Can you work these out from the model? Positions are in its coordinate system, mm. A direction names the side the tool comes from. Coordinates: 2 decimals unless noted, no trailing zeros. Order: outer loops, then holes, each group sorted by start corner. A loop starts at its lowest first (then second) coordinate and runs counter-clockwise, first axis right, second up. Notation, with made-up numbers: (-3, 5) -> (8, 5) arc R6 ccw to (8, 13) -> close; hole circle Ø3 at (51.25, -34.75). An arc over 180 degrees is marked (long way). Write item = value, one per line.
Autodesk Inventor part; units mm, degrees
ref_plane "YZ Plane" through (0, 0, 0) normal (1, 0, 0) x (0, 1, 0)
ref_plane "XZ Plane" through (0, 0, 0) normal (0, 1, 0) x (-1, 0, 0)
ref_plane "XY Plane" through (0, 0, 0) normal (0, 0, 1) x (1, 0, 0)
sketch "Base" plane through (0, 0, 0) normal (0, 1, 0) x (-1, 0, 0)
  line L0 (0, 0) -> (-12, 0)
  line L1 (-12, 0) -> (-12, -11.4)
  line L2 (-12, -11.4) -> (0, -11.4) construction
  line L3 (0, -11.4) -> (0, 0)
  circle A0 centre (-3.175, -3.175) radius 3.175
  circle A1 centre (-6.5, -11.4) radius 6.5
  line L4 (-6.5, -4.9) -> (-6.5, 0)
  line L5 (-6.5, -4.9) -> (-12, -4.9)
  line L6 (-9.25, -4.9) -> (-9.25, 0)
  point P0 (0, 0)
  point P1 (-12, -7.9359)
  dimension "d24" = 13
  dimension "d21" = 12
  dimension "d22" = 11.4
  dimension "d23" = 6.35
  dimension "d26" = 5.5
  dimension "d36" = 5.5
extrude "Stock" add sketch "Base" against normal blind 19 contours L4 L5 L6 L0 | L0 A0 A1 L4 | L0 L3 A0 | A0 A1 | L3 A1 A0 picked at (-3.3154, -3.7047)
hole "3mm Hole" at (3.175, 0, -3.175) direction (0, -1, 0) diameter 3.2004 end through all
equation "\"d36\" = d26"
properties part number "Joint Spacer" material "Aluminum 6061"
Item 1: If I drill on probe 1 along Z at (x, y) = (8.5, -12.5); probe 2 along Z at (x, y) = (3.25, -13.25); probe 3 along Z at (x, y) = (4.25, -1.5), over which ranges is the centre line in solid material (lowest first)?
A:
probe_1 = -4.9 to 0
probe_2 = -5.77 to -4.77, -1.58 to 0
probe_3 = -5.3 to -4.36, -1.99 to 0
Item 2: I want a section at B-B, the plane x = 7.5. Please give me the cut outline in (y, z), plus the area to 3 significant figures.
A:
outline = (-19, -4.9) -> (0, -4.9) -> (0, 0) -> (-19, 0) -> close
area = 93.1 mm2
Item 3: For faces 5 (the flat face through (5, -19, -2)), 6 (the flat face through (8, -9, -4.9)), which set-ups out of +Z, -Z, +X, -X, +Y, -Y let a thin tool reach every point of the face, with its end or its side?
A:
face_5 = +Z, -Z, +X, -X, -Y
face_6 = -Z, +X, +Y, -Y
Item 4: If we mould it in two halves opening along X, with no side actions, what happens to faces 1 (the flat face through (5, -9, 0)), 2 (the flat face through (9.25, -9, -2)), 3 (the cylindrical face through (4.149, -9.633, -4.445)), 4 (the flat face through (0, -9, -6))? For each: pulls with the +X half, pulls with the -X half, needs draft (parallel to the pull), parting line crosses it, or undercut.
A:
face_1 = needs draft
face_2 = pulls with the +X half
face_3 = undercut
face_4 = pulls with the -X half
Item 5: I'm going to push flat-ended pins straight in: P1, Ø2, axis at x = 8, y = -9, coming from the -Z side; P2, Ø1, axis at y = -4, z = -10, coming from the +X side; P3, Ø1, axis at y = -11, z = -8, coming from the +X side. Where does each tip first touch, or does it pass through?
A:
P1 = -4.9
P2 = 0.28
P3 = 1.3
Item 6: I want a section at A-A, the plane z = -2.5. Please give me the cut outline in (x, y).
A:
outline = (0, -19) -> (1.72, -19) -> (1.72, 0) -> (0, 0) -> close; (4.63, -19) -> (9.25, -19) -> (9.25, 0) -> (4.63, 0) -> close
Item 7: I want a section at C-C, the plane y = -15. Please give me the cut outline in (x, z) (3 decimals).
A:
outline = (0, -11.4) arc R6.5 cw to (6.5, -4.9) -> (9.25, -4.9) -> (9.25, 0) -> (0, 0) -> close; hole circle Ø3.2 at (3.175, -3.175)
Item 8: I want a section at D-D, the plane z = -7.25. Please give me the cut outline in (x, y).
A:
outline = (0, -19) -> (1.5, -19) -> (1.5, 0) -> (0, 0) -> close
